Could you check a few things on this model? Use its own coordinates, in mm. A direction names the side the tool comes from. Give positions to 0.01 mm unless a question says otherwise; leave off trailing zeros. Order: outer loops, then holes, each group sorted by start corner. A loop starts at its lowest first (then second) coordinate and runs counter-clockwise, first axis right, second up. Notation, with made-up numbers: M 33.5,88 L 79.5,88 A25 ccw 79.5,103 Z; hole C -8,-23.5 d10. An arc over 180 degrees is marked long. Return JSON: item names as keys, results as strings. Group by question number.
```python
from build123d import *

# Parameters (mm, degrees)
F1_DEPTH = 50.8
F2_W     = 55.813026
F2_H     = 50.985549
F3_DEPTH = 0.508


with BuildPart() as f1:
    # F0 (on Right) → F1 (new body)
    with BuildSketch(Plane.YZ):
        Polygon((-23.537235, 56.615818), (-22.788359, 0), (23.725847, 0), (23.725847, 127.323955), (-67.180149, 71.632735), (-43.716218, 46.760969), align=None)
    extrude(amount=-F1_DEPTH)

    # F2 (on Top) → F3 (join)
    with BuildSketch(Plane.XY):
        with Locations((-25.752099, 0.632371)):
            Rectangle(F2_W, F2_H)
    extrude(amount=-F3_DEPTH)


solid = f1.part
```
1. I need wall thicknesses on L1, parallel to X at y = -3, z = 42; L2, parallel to Z at x = 0.5, y = 20; L3, parallel to Z at x = -13, y = -52.5. Which ranges of each line are inside material? Lowest first, please. Write a range as from..to.
2. If we mould it in two halves opening along Z, with no side actions, what happens to faces 1 (the flat face through (-28, -24, 0)), 2 (the flat face through (-26, 1, -0.508)), 3 (the flat face through (0, -12, 65))? For each: pulls with the +Z half, pulls with the -Z half, needs draft (parallel to the pull), parting line crosses it, or undercut.
3. Imagine slicing it at B-B, the plane x = -2.5. Please give me the cut outline in (y, z).
4. Imagine slicing it at D-D, the plane y = -5. Please give me the cut outline in (x, z), plus the area to 3 significant figures.
5. Imagine slicing it at C-C, the plane y = -17.5. Please give me the cut outline in (x, z), plus the area to 3 significant figures.
6. Imagine slicing it at A-A, the plane z = 53. Please give me the cut outline in (x, y).
7. For pin 1 (6 mm diameter, centred on x = -36.5, y = -43, fed in from +Z); pin 2 (1.5 mm diameter, centred on x = -38.5, z = 87.5, fed in from -Y); pin 3 (2 mm diameter, centred on x = -5.5, y = -38.5, fed in from -Z), each with a flat end and sliding along its axis, tell me the tip position at first contact or that it passes through.
8. Which directions (+Z, -Z, +X, -X, +Y, -Y) give clear straight access to the entire face, cutting with the end or side of a thin tool? Please do faces 4 (the flat face through (-25, 23.726, 63)), 5 (the flat face through (-50.8, -12, 65)), 6 (the flat face through (-25.04, -55.61, 59.37)).
Values:
{
 "1": {"L1": "x = -50.8..0", "L2": "z = -0.51..0", "L3": "z = 56.07..80.63"},
 "2": {"face 1": "undercut", "face 2": "pulls with the -Z half", "face 3": "needs draft"},
 "3": {"outline": "M -67.18,71.63 L -43.72,46.76 L -23.54,56.62 L -22.79,0 L -24.86,0 L -24.86,-0.51 L 26.13,-0.51 L 26.13,0 L 23.73,0 L 23.73,127.32 Z"},
 "4": {"outline": "M -53.66,-0.51 L 2.15,-0.51 L 2.15,0 L 0,0 L 0,109.73 L -50.8,109.73 L -50.8,0 L -53.66,0 Z", "area": "5,600 mm²"},
 "5": {"outline": "M -53.66,-0.51 L 2.15,-0.51 L 2.15,0 L 0,0 L 0,102.07 L -50.8,102.07 L -50.8,0 L -53.66,0 Z", "area": "5,210 mm²"},
 "6": {"outline": "M -50.8,-49.6 L 0,-49.6 L 0,-30.94 L -50.8,-30.94 Z; M -50.8,-23.49 L 0,-23.49 L 0,23.73 L -50.8,23.73 Z"},
 "7": {"pin 1": "stops at z = 88.28", "pin 2": "stops at y = -42.5", "pin 3": "stops at z = 48.82"},
 "8": {"face 4": "+Z, +X, -X, +Y", "face 5": "+Z, -X, +Y, -Y", "face 6": "-Z, +X, -X, -Y"}
}
